Verification items for this drawing (mm, ordinates from the low corner). A direction names the side the tool comes from. Give positions to 0.01 mm unless a question says otherwise; leave off trailing zeros. Write each loop counter-clockwise with the first axis right and the second up, starting at its lowest first coordinate (ties: lowest second). Pieces come first, ordered by that corner, then holes. Notation, with made-up numbers: M 60,-3 L 74,-3 A15 ccw 74,22 Z; hole C 46.5,-28.5 d1. An arc over 180 degrees is marked long. Use one line per item in the form item = value. Start each with the question number.
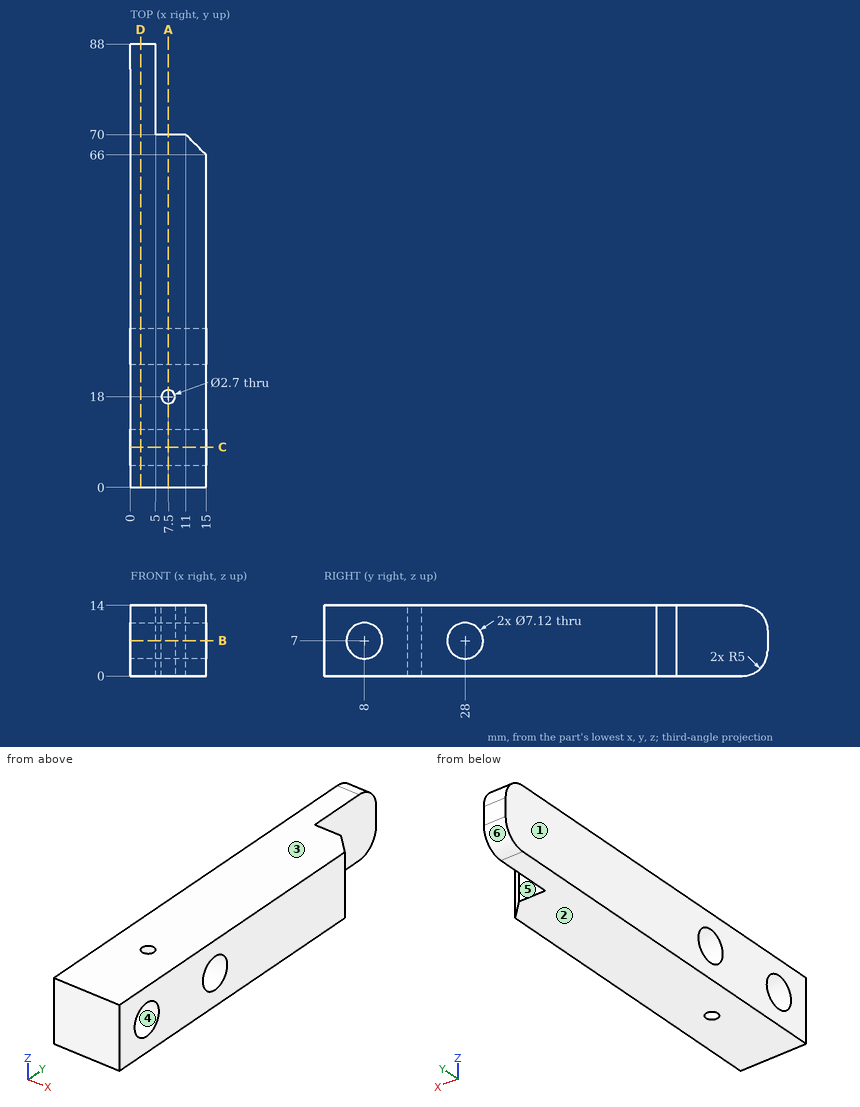
(1) Sectioned sample at C-C, the plane y = 8. Record the boundary of the cut face in (x, z).
(2) Depth check by flat-ended pin: pin 1 (5 mm diameter, centred on x = 9.5, z = 6.5, fed in from +Y). Enter the tip coordinate at first touch or a pass-through.
(3) Tool access check on the marked faces 5 and 6. Record the directions out of +Z, -Z, +X, -X, +Y, -Y that give a thin tool (end or side, any length) a straight path to the whole face; none if there is none.
(4) Sectioned sample at A-A, the plane x = 7.5. Record the boundary of the cut face in (y, z), plus the area to 3 significant figures.
(5) Sectioned sample at B-B, the plane z = 7. Record the boundary of the cut face in (x, y).
(6) Thickness scan on probe 1 along Y at (x, z) = (10.5, 7); probe 2 along Y at (x, z) = (4.25, 7); probe 3 along Y at (x, z) = (7.5, 4.75). Record the ranges inside material, lowest first. Write a range as [from, to].
(7) Draft check along Z on the marked faces 1, 2, 3 and 4. Enter one of: released by +Z, released by -Z, zero draft, split by the parting line, or undercut.
(8) Sectioned sample at D-D, the plane x = 2. Record the boundary of the cut face in (y, z), plus the area to 3 significant figures.
Numbers:
q1.outline = M 0,0 L 15,0 L 15,3.44 L 0,3.44 Z; M 0,10.56 L 15,10.56 L 15,14 L 0,14 Z
q2.pin_1 = 70
q3.face_5 = +Z, -Z, +X, +Y
q3.face_6 = -Z, +X, -X, +Y
q4.outline = M 0,0 L 16.65,0 L 16.65,14 L 0,14 Z; M 19.35,0 L 70,0 L 70,14 L 19.35,14 Z; hole C 8,7 d7.12; hole C 28,7 d7.12
q4.area = 863 mm2
q5.outline = M 0,0 L 15,0 L 15,4.44 L 0,4.44 Z; M 0,11.56 L 15,11.56 L 15,24.44 L 0,24.44 Z; M 0,31.56 L 15,31.56 L 15,66 L 11,70 L 5,70 L 5,88 L 0,88 Z; hole C 7.5,18 d2.7
q6.probe_1 = [0, 4.44], [11.56, 24.44], [31.56, 70]
q6.probe_2 = [0, 4.44], [11.56, 24.44], [31.56, 88]
q6.probe_3 = [0, 5.24], [10.76, 16.65], [19.35, 25.24], [30.76, 70]
q7.face_1 = zero draft
q7.face_2 = released by -Z
q7.face_3 = released by +Z
q7.face_4 = undercut
q8.outline = M 0,0 L 83,0 A5 ccw 88,5 L 88,9 A5 ccw 83,14 L 0,14 Z; hole C 8,7 d7.12; hole C 28,7 d7.12
q8.area = 1,140 mm2
